from build123d import *

# Parameters (mm, degrees)
SKETCH1_R           = 6.55
BOSS_EXTRUDE1_DEPTH = 11.5
SKETCH9_W           = 19
SKETCH9_H           = 30
CUT_EXTRUDE4_DEPTH  = 45.25
SKETCH12_W          = 63.5
SKETCH12_H          = 9
BOSS_EXTRUDE2_DEPTH = 25
CUT_EXTRUDE5_DEPTH  = 80


with BuildPart() as part:
    # Sketch1 → Boss-Extrude1 (new body, symmetric)
    with BuildSketch(Plane.XY):
        Polygon((-12.5, -58), (-31.75, -58), (-31.75, -67), (31.75, -67), (31.75, -58), (12.5, -58), (12.5, 12), (-12.5, 12), align=None)
        Circle(SKETCH1_R, mode=Mode.SUBTRACT)
    extrude(amount=BOSS_EXTRUDE1_DEPTH, both=True)

    # Sketch9 → Cut-Extrude4 (cut, through all)
    with BuildSketch(Plane.ZY.offset(12.5)):
        with Locations((2, -3)):
            Rectangle(SKETCH9_W, SKETCH9_H)
    extrude(amount=-CUT_EXTRUDE4_DEPTH, mode=Mode.SUBTRACT)

    # Sketch12 → Boss-Extrude2 (add)
    with BuildSketch(Plane.XY.offset(11.5)):
        with Locations((0, -62.5)):
            Rectangle(SKETCH12_W, SKETCH12_H)
    extrude(amount=BOSS_EXTRUDE2_DEPTH)

    # Sketch11 → Cut-Extrude5 (cut, through all)
    with BuildSketch(Plane.XZ.offset(67)):
        with BuildLine():
            Line((-21.9, 29.5), (-21.9, -4.5))
            ThreePointArc((-21.9, -4.5), (-25.4, -8), (-28.9, -4.5))
            Line((-28.9, -4.5), (-28.9, 29.5))
            ThreePointArc((-28.9, 29.5), (-25.4, 33), (-21.9, 29.5))
        make_face()
        with BuildLine():
            Line((21.9, -4.5), (21.9, 29.5))
            ThreePointArc((21.9, 29.5), (25.4, 33), (28.9, 29.5))
            Line((28.9, 29.5), (28.9, -4.5))
            ThreePointArc((28.9, -4.5), (25.4, -8), (21.9, -4.5))
        make_face()
    extrude(amount=-CUT_EXTRUDE5_DEPTH, mode=Mode.SUBTRACT)


solid = part.part
Read the model definition and answer for the solid it produces. Units are mm, in the model's axes. A direction names the side the tool comes from. Give positions to 0.01 mm unless a question says otherwise; leave off trailing zeros. Write each loop counter-clockwise with the first axis right and the second up, starting at its lowest first coordinate (ties: lowest second). Pieces come first, ordered by that corner, then holes. Notation, with made-up numbers: (68, -29.5) - (111, -29.5) arc R11 ccw to (111, -14.5) - close; hole circle Ø11 at (17, 65). An arc over 180 degrees is marked (long way). Answer in a Markdown table with one row per item. Add a question column.
Item 1: Section C-C, the plane x = -25.4 is taken. Write down the section's boundary in (y, z), and give its area (3 significant figures).
Item 2: Find the intervals of material crossed by L1, parallel to X at y = -62.5, z = 2; L2, parallel to Y at x = 0, z = -9; L3, parallel to X at y = 0, z = -9, in increasing order.
Item 3: Section B-B, the plane y = 0 is taken. Write down the section's boundary in (x, z), and give its area (3 significant figures).
Item 4: Section D-D, the plane z = 8 is taken. Write down the section's boundary in (x, y).
Item 5: Determine the mould class of faces 4 (the face through (-28.9, -63, 12)), 5 (the face through (31.75, -63, 12)), 6 (the face through (0, -62, 36.5)) for opening direction X: pulls with the +X half, pulls with the -X half, needs draft (parallel to the pull), parting line crosses it, or undercut.
Item 6: A tool of negligible diameter and unlimited length cuts with its end or side. For faces 1 (the face through (-25.3, -62.6, -8)), 2 (the face through (12.5, -31, -2)), 3 (the face through (0, -38, 11.5)), from which of +Z, -Z, +X, -X, +Y, -Y can it reach the whole face along a straight path? Write none if from no direction.
Item 7: Section A-A, the plane z = 27.5 is taken. Write down the section's boundary in (x, y), and give its area (4 significant figures).
Item 8: Flat-ended cylindrical pins translate along their axes: P1, Ø20, axis at x = -6, y = 4, coming from the +Z side; P2, Ø5, axis at y = -17.5, z = -2, coming from the +X side; P3, Ø12, axis at y = -40, z = 10.5, coming from the -X side. Find the tip coordinate at first contact, or state that the pin passes through.
Recorded:
| question | item | result |
|---|---|---|
| 1 | outline | (-67, -11.5) - (-58, -11.5) - (-58, -8) - (-67, -8) - close; (-67, 33) - (-58, 33) - (-58, 36.5) - (-67, 36.5) - close |
| 1 | area | 63.0 mm2 |
| 2 | L1 | x = -31.75 to -28.9, -21.9 to 21.9, 28.9 to 31.75 |
| 2 | L2 | y = -67 to -6.55, 6.55 to 12 |
| 2 | L3 | x = -12.5 to -6.55, 6.55 to 12.5 |
| 3 | outline | (-12.5, -11.5) - (-6.55, -11.5) - (-6.55, -7.5) - (-12.5, -7.5) - close; (6.55, -11.5) - (12.5, -11.5) - (12.5, -7.5) - (6.55, -7.5) - close |
| 3 | area | 47.6 mm2 |
| 4 | outline | (-31.75, -67) - (-28.9, -67) - (-28.9, -58) - (-31.75, -58) - close; (-21.9, -67) - (21.9, -67) - (21.9, -58) - (12.5, -58) - (12.5, -18) - (-12.5, -18) - (-12.5, -58) - (-21.9, -58) - close; (28.9, -67) - (31.75, -67) - (31.75, -58) - (28.9, -58) - close |
| 5 | face 4 | undercut |
| 5 | face 5 | pulls with the +X half |
| 5 | face 6 | needs draft |
| 6 | face 1 | +Y, -Y |
| 6 | face 2 | +Z, -Z, +X, +Y |
| 6 | face 3 | +Z, +X, -X, +Y |
| 7 | outline | (-31.75, -67) - (-28.9, -67) - (-28.9, -58) - (-31.75, -58) - close; (-21.9, -67) - (21.9, -67) - (21.9, -58) - (-21.9, -58) - close; (28.9, -67) - (31.75, -67) - (31.75, -58) - (28.9, -58) - close |
| 7 | area | 445.5 mm2 |
| 8 | P1 | stops at z = -7.5 |
| 8 | P2 | stops at x = 12.5 |
| 8 | P3 | stops at x = -12.5 |
